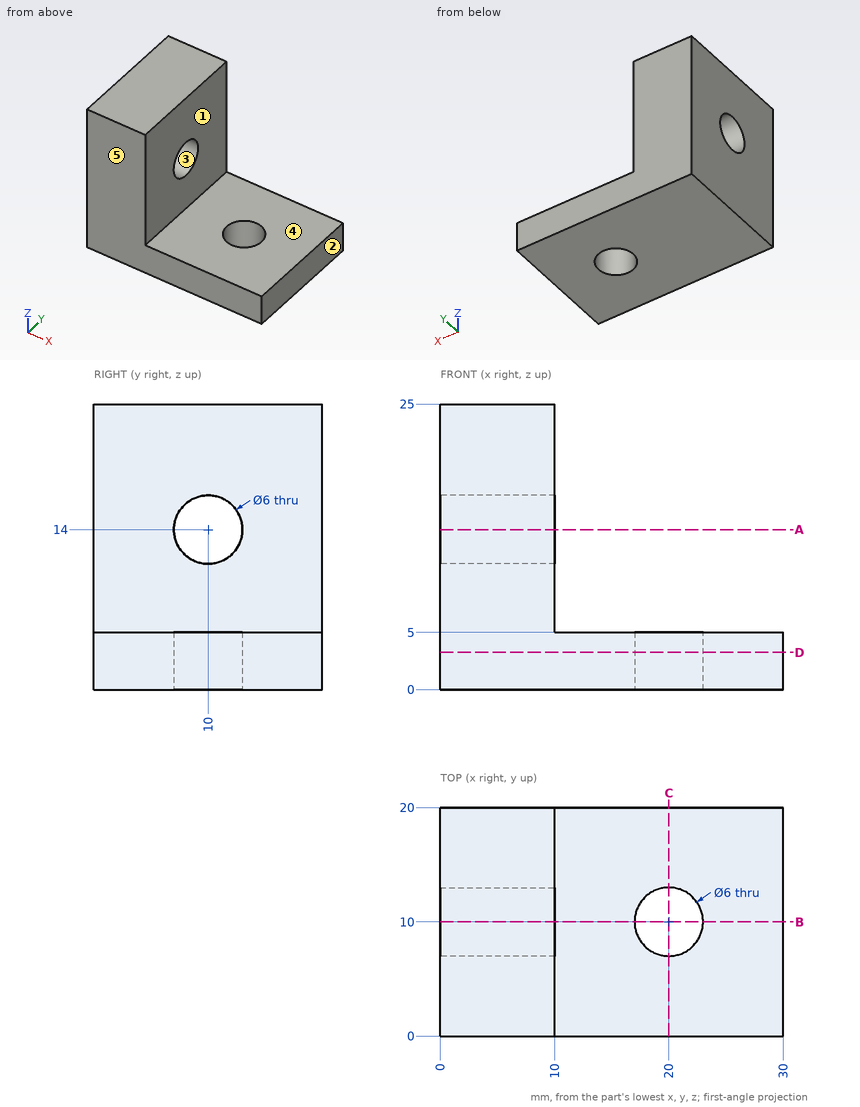
Design review of the part shown in the three views and the two pictorial views. Dimensions are in mm from the part's minimum x, y and z. A direction names the side the tool comes from. Round coordinates to 2 decimals unless told otherwise and drop trailing zeros. Write each loop counter-clockwise with the first axis right and the second up, starting at its lowest first coordinate (ties: lowest second). Pieces come first, ordered by that corner, then holes.
Item 1: Consider section A-A on z = 14. Give the boundary of the cut face in (x, y), and give its area (3 significant figures).
Item 2: For the marked faces 1 and 2, list the 3-axis set-ups (+Z, -Z, +X, -X, +Y, -Y) from which the entire face can be reached by the end or side of a thin tool; tool diameter is ignored.
Item 3: Consider section B-B on y = 10. Give the boundary of the cut face in (x, z).
Item 4: For pin 1 Ø4 at (y, z) = (15.5, 9.5) entering from +X; pin 2 Ø8 at (x, y) = (20, 10) entering from -Z; pin 3 Ø1 at (x, y) = (26.5, 14) entering from +Z, all flat-tipped, find the tip position at first contact; note any pin that passes through.
Item 5: Consider section D-D on z = 3.25. Give the boundary of the cut face in (x, y), and give its area (3 significant figures).
Item 6: Consider section C-C on x = 20. Give the boundary of the cut face in (y, z), and give its area (3 significant figures).
Item 7: Wall thickness on L1, parallel to Y at x = 4, z = 14; L2, parallel to Z at x = 5.75, y = 10; L3, parallel to Z at x = 15.75, y = 12.5: over which ranges is each line inside the solid? List them lowest first.
Item 8: Draft analysis for pull direction Y (two halves, no side actions). For the marked faces 3, 4 and 5, state which applies: released by +Y, released by -Y, zero draft, split by the parting line, or undercut.
Check values:
1. outline: (0, 0) - (10, 0) - (10, 7) - (0, 7) - close; (0, 13) - (10, 13) - (10, 20) - (0, 20) - close
1. area: 140 mm2
2. face 1: +Z, +X, +Y, -Y
2. face 2: +Z, -Z, +X, +Y, -Y
3. outline: (0, 0) - (17, 0) - (17, 5) - (10, 5) - (10, 11) - (0, 11) - close; (0, 17) - (10, 17) - (10, 25) - (0, 25) - close; (23, 0) - (30, 0) - (30, 5) - (23, 5) - close
4. pin 1: stops at x = 10
4. pin 2: stops at z = 0
4. pin 3: stops at z = 5
5. outline: (0, 0) - (30, 0) - (30, 20) - (0, 20) - close; hole circle Ø6 at (20, 10)
5. area: 572 mm2
6. outline: (0, 0) - (7, 0) - (7, 5) - (0, 5) - close; (13, 0) - (20, 0) - (20, 5) - (13, 5) - close
6. area: 70.0 mm2
7. L1: y = 0 to 7, 13 to 20
7. L2: z = 0 to 11, 17 to 25
7. L3: z = 0 to 5
8. face 3: undercut
8. face 4: zero draft
8. face 5: released by -Y
